Design review of the part built by this model. Coordinates are the model's own, in mm. A direction names the side the tool comes from. Coordinates: 2 decimals unless noted, no trailing zeros. One line per question, with ' | ' between items.
from build123d import *

# Parameters (mm, degrees)
SKETCH1_R                   = 27.559
BOSS_EXTRUDE1_DEPTH         = 4.7625
SKETCH2_R                   = 1.61925
F_40_0_098_DIAMETER_HOLE1_D = 2.4892
CUT_EXTRUDE1_DEPTH          = 40.264212309
SKETCH9_R                   = 2.3622
CUT_EXTRUDE2_DEPTH          = 2.54


with BuildPart() as part:
    # Sketch1 → Boss-Extrude1 (new body)
    with BuildSketch(Plane(origin=(0, 0, 0), x_dir=(1, 0, 0), z_dir=(0, 1, 0))):
        with Locations(Location((0, 0, 0), (0, 0, 270))):
            Circle(SKETCH1_R)
    extrude(amount=BOSS_EXTRUDE1_DEPTH)

    # Cut-Sweep1: sweep along a curve in space
    with BuildLine() as cut_sweep1_path:
        ThreePointArc((0, 0, 27.559), (19.487155783, 0, 19.487155783), (27.559, 0, 0))
        ThreePointArc((27.559, 0, 0), (19.487155783, 0, -19.487155783), (0, 0, -27.559))
        ThreePointArc((0, 0, -27.559), (-19.487155783, 0, -19.487155783), (-27.559, 0, 0))
        ThreePointArc((-27.559, 0, 0), (-19.487155783, 0, 19.487155783), (0, 0, 27.559))
    # Sketch2 → Cut-Sweep1 (sweep, cut)
    with BuildSketch(Plane.XY):
        with Locations((-27.559, 2.38125)):
            Circle(SKETCH2_R)
    sweep(path=cut_sweep1_path.line, mode=Mode.SUBTRACT)

    # #40 (0.098) Diameter Hole1 (through all)
    with Locations(Plane(origin=(0, 0, 0), x_dir=(0, 0, -1), z_dir=(0, -1, 0))):
        with Locations((0, 0)):
            Hole(F_40_0_098_DIAMETER_HOLE1_D / 2)

    # Sketch7 → Cut-Extrude1 (cut, through all)
    with BuildSketch(Plane(origin=(0, 4.7625, 0), x_dir=(1, 0, 0), z_dir=(0, 1, 0))):
        with BuildLine():
            ThreePointArc((-2.2225, 3.84948292), (-0.77186615, 4.377470462), (0.77186615, 4.377470462))
            ThreePointArc((0.77186615, 4.377470462), (9.824364413, 11.765183037), (21.41292145, 10.271406718))
            ThreePointArc((21.41292145, 10.271406718), (16.608536278, 16.975615562), (9.800916515, 21.632314635))
            ThreePointArc((9.800916515, 21.632314635), (-0.036614117, 15.327632806), (-2.2225, 3.84948292))
        make_face()
        with BuildLine():
            ThreePointArc((2.2225, 3.84948292), (3.40506755, 2.857190925), (4.176933699, 1.520279537))
            ThreePointArc((4.176933699, 1.520279537), (15.101129597, -2.625557639), (19.601759876, -13.408430586))
            ThreePointArc((19.601759876, -13.408430586), (22.688512471, -7.017578133), (23.749, 0))
            ThreePointArc((23.749, 0), (23.720380824, 1.1655619), (23.634592274, 2.328314635))
            ThreePointArc((23.634592274, 2.328314635), (13.255812331, 7.695525158), (2.2225, 3.84948292))
        make_face()
        with BuildLine():
            ThreePointArc((13.833675759, -19.304), (13.292426448, -7.632107648), (4.445, 0))
            ThreePointArc((4.445, 0), (4.176933699, -1.520279537), (3.40506755, -2.857190925))
            ThreePointArc((3.40506755, -2.857190925), (5.276765184, -14.390740676), (-1.811161574, -23.679837304))
            ThreePointArc((-1.811161574, -23.679837304), (6.397046182, -22.871222117), (13.833675759, -19.304))
        make_face()
        with BuildLine():
            ThreePointArc((-9.800916515, -21.632314635), (0.036614117, -15.327632806), (2.2225, -3.84948292))
            ThreePointArc((2.2225, -3.84948292), (0.77186615, -4.377470462), (-0.77186615, -4.377470462))
            ThreePointArc((-0.77186615, -4.377470462), (-9.824364413, -11.765183037), (-21.41292145, -10.271406718))
            ThreePointArc((-21.41292145, -10.271406718), (-16.608536278, -16.975615562), (-9.800916515, -21.632314635))
        make_face()
        with BuildLine():
            ThreePointArc((-23.634592274, -2.328314635), (-13.255812331, -7.695525158), (-2.2225, -3.84948292))
            ThreePointArc((-2.2225, -3.84948292), (-3.40506755, -2.857190925), (-4.176933699, -1.520279537))
            ThreePointArc((-4.176933699, -1.520279537), (-15.101129597, 2.625557639), (-19.601759876, 13.408430586))
            ThreePointArc((-19.601759876, 13.408430586), (-23.00558246, 5.895606556), (-23.634592274, -2.328314635))
        make_face()
        with BuildLine():
            ThreePointArc((-4.445, 0), (-4.176933699, 1.520279537), (-3.40506755, 2.857190925))
            ThreePointArc((-3.40506755, 2.857190925), (-5.276765184, 14.390740676), (1.811161574, 23.679837304))
            ThreePointArc((1.811161574, 23.679837304), (-6.397046182, 22.871222117), (-13.833675759, 19.304))
            ThreePointArc((-13.833675759, 19.304), (-13.292426448, 7.632107648), (-4.445, 0))
        make_face()
    extrude(amount=-CUT_EXTRUDE1_DEPTH, mode=Mode.SUBTRACT)

    # Sketch9 → Cut-Extrude2 (cut)
    with BuildSketch(Plane(origin=(0, 4.7625, 0), x_dir=(1, 0, 0), z_dir=(0, 1, 0))):
        with Locations(Location((0, 0, 0), (0, 0, 270))):
            Circle(SKETCH9_R)
    extrude(amount=-CUT_EXTRUDE2_DEPTH, mode=Mode.SUBTRACT)


solid = part.part
Q1. Draft analysis for pull direction X (two halves, no side actions). For faces 1 (the flat face through (-6, 4.762, 0)), 2 (the cylindrical face through (16.691, 2.415, -16.894)), 3 (the cylindrical face through (-26.904, 0.376, -5.974)), 4 (the cylindrical face through (-3.391, 2.415, 2.874)), state which applies: +X half, -X half, draft (parallel to the pull), parting line (faces both ways), or undercut.
Returned:
face 1: draft | face 2: undercut | face 3: parting line | face 4: undercut
Q2. Take a section at A-A (z = -9.5). State how many separate pieces and enclosed holes the cut face has, plus the area to 3 significant figures.
Returned:
separate pieces: 4 | enclosed holes: 0 | area: 149 mm²
Q3. For pin 1 (4 mm diameter, centred on x = 0, z = 0.5, fed in from +Y); pin 2 (1 mm diameter, centred on y = 1.5, z = 10.5, fed in from +X); pin 3 (2 mm diameter, centred on x = 4.5, y = 0.5, fed in from -Z); pin 4 (1.5 mm diameter, centred on x = 21, z = 20.5, fed in from -Y), all flat-tipped, find the tip position at first contact; note any pin that passes through.
Returned:
pin 1: stops at y = 4.76 | pin 2: stops at x = 24.59 | pin 3: stops at z = -27.34 | pin 4: passes through
Q4. To check wall thickness, follow line 1 along X through (y, z) = (1.05, 11); line 2 along Z through (x, y) = (-16, 4.2); line 3 along X through (y, z) = (4.1, -19). State the ranges of each line that lie inside material, in increasing order.
Returned:
line 1: x = -24.26 to -21.05, -20.02 to -7.75, 2.03 to 5.72, 14.45 to 19.43, 21.05 to 24.26 | line 2: z = -22.44 to -3.58, 7.24 to 12.18, 17.55 to 22.44 | line 3: x = -19.96 to -13.94, -3.24 to 3.51, 14.25 to 19.96
Q5. Tool access review of faces 5 (the cylindrical face through (0.37, 1.13, 1.19)), 6 (the flat face through (-1, 2.222, 1)): name each direction out of +Z, -Z, +X, -X, +Y, -Y from which nothing blocks a thin tool from reaching the whole face with its end or side.
Returned:
face 5: +Y, -Y | face 6: +Y
